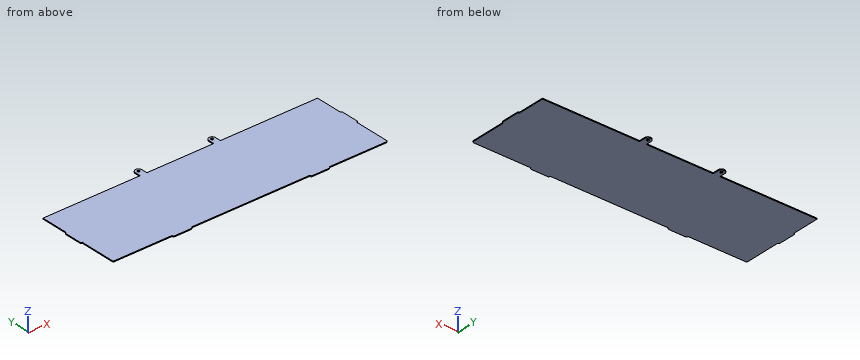
from build123d import *

# Parameters (mm, degrees)
SKETCH1_R           = 2.38125
BOSS_EXTRUDE1_DEPTH = 0.88392
FILLET1_R           = 2.54


with BuildPart() as part:
    # Sketch1 → Boss-Extrude1 (new, symmetric)
    with BuildSketch(Plane.XY):
        with BuildLine():
            Line((-260.731250444, 160.9598), (-76.2, 160.9598))
            Line((-76.2, 160.9598), (-76.2, 172.0723))
            ThreePointArc((-76.2, 172.0723), (-69.85, 178.4223), (-63.5, 172.0723))
            Line((-63.5, 172.0723), (-63.5, 160.9598))
            Line((-63.5, 160.9598), (63.5, 160.9598))
            Line((63.5, 160.9598), (63.5, 172.0723))
            ThreePointArc((63.5, 172.0723), (69.85, 178.4223), (76.2, 172.0723))
            Line((76.2, 172.0723), (76.2, 160.9598))
            Line((76.2, 160.9598), (260.731250444, 160.9598))
            Line((260.731250444, 160.9598), (260.731250444, 109.36605))
            Line((260.731250444, 109.36605), (263.271250444, 109.36605))
            Line((263.271250444, 109.36605), (263.271250444, 72.85355))
            Line((263.271250444, 72.85355), (260.731250444, 72.85355))
            Line((260.731250444, 72.85355), (260.731250444, 3.00355))
            Line((260.731250444, 3.00355), (149.018750222, 3.00355))
            Line((149.018750222, 3.00355), (149.018750222, 0))
            Line((149.018750222, 0), (112.506250222, 0))
            Line((112.506250222, 0), (112.506250222, 3.00355))
            Line((112.506250222, 3.00355), (-112.506250222, 3.00355))
            Line((-112.506250222, 3.00355), (-112.506250222, 0))
            Line((-112.506250222, 0), (-149.018750222, 0))
            Line((-149.018750222, 0), (-149.018750222, 3.00355))
            Line((-149.018750222, 3.00355), (-260.731250444, 3.00355))
            Line((-260.731250444, 3.00355), (-260.731250444, 72.85355))
            Line((-260.731250444, 72.85355), (-263.271250444, 72.85355))
            Line((-263.271250444, 72.85355), (-263.271250444, 109.36605))
            Line((-263.271250444, 109.36605), (-260.731250444, 109.36605))
            Line((-260.731250444, 109.36605), (-260.731250444, 160.9598))
        make_face()
        with Locations(Location((-69.85, 172.0723, 0), (0, 0, 180))):
            Circle(SKETCH1_R, mode=Mode.SUBTRACT)
        with Locations(Location((69.85, 172.0723, 0), (0, 0, 180))):
            Circle(SKETCH1_R, mode=Mode.SUBTRACT)
    extrude(amount=BOSS_EXTRUDE1_DEPTH, both=True)

    # Fillet1
    fillet1_edges = [part.edges().sort_by_distance(p)[0] for p in [
        (-263.271250444, 109.36605, 0),
        (-263.271250444, 72.85355, 0),
        (263.271250444, 109.36605, 0),
        (263.271250444, 72.85355, 0),
        (149.018750222, 0, 0),
        (112.506250222, 0, 0),
        (-112.506250222, 0, 0),
        (-149.018750222, 0, 0),
        (-260.731250444, 3.00355, 0),
        (260.731250444, 3.00355, 0),
    ]]
    fillet(fillet1_edges, radius=FILLET1_R - 0.0001)  # a hair under: the kernel refuses the full size


solid = part.part
Here's how the part is built. I have some questions about the finished solid (model axes, mm). Coordinates: 2 decimals unless noted, no trailing zeros. Order: outer loops, then holes, each group sorted by start corner. A loop starts at its lowest first (then second) coordinate and runs counter-clockwise, first axis right, second up.
Item 1: For P1, Ø1, axis at y = 116.5, z = 0, coming from the +X side; P2, Ø0.5, axis at x = -188, z = 0.5, coming from the -Y side; P3, Ø0.9, axis at y = 164.5, z = 0, coming from the -X side, each with a flat end and sliding along its axis, tell me the tip position at first contact or that it passes through.
Result sheet:
P1: stops at x = 260.73
P2: stops at y = 3
P3: stops at x = -76.2
Item 2: If we section it at A-A on z = -0.2: State how many separate pieces and enclosed holes the cut face has, plus the area to 3 significant figures.
Result sheet:
separate pieces: 1
enclosed holes: 2
area: 83,100 mm2
Item 3: If we section it at B-B on x = -89.5: List the corners of the cut face in (y, z) for me.
Result sheet:
outline: (3, -0.88) - (160.96, -0.88) - (160.96, 0.88) - (3, 0.88) - close
Item 4: I need wall thicknesses on line 1 (Y direction, x = -69.85, z = -0.2); line 2 (Y direction, x = 106, z = 0.25); line 3 (X direction, y = 141, z = 0.35). Which ranges of each line are inside material? Lowest first, please.
Result sheet:
line 1: y = 3 to 169.69, 174.45 to 178.42
line 2: y = 3 to 160.96
line 3: x = -260.73 to 260.73
